Design review of the part built by this model. Coordinates are the model's own, in mm. Face numbers are marked on the shaded views. A direction names the side the tool comes from. Coordinates: 2 decimals unless noted, no trailing zeros. Loops run counter-clockwise (first coordinate to the right, second up) from the corner with the lowest first, then second, coordinate; pieces in that order, holes last. Notation, with made-up numbers: M 36,-38.75 L 77,-38.75 A30 cw 77,-1.75 Z; hole C -36,70.25 d8. An arc over 180 degrees is marked long. Answer as a JSON object with one key per item and string values. Group by question number.
1. Machinability: for the marked faces 5, 6, 7, 8 and 9, which of the approach directions +Z, -Z, +X, -X, +Y, -Y give a long, thin tool a straight path to every point of the face, cutting with its end or side? Answer none if there is none.
2. Consider section D-D (y = 7.75). State the section outline as (x, z) points, then the cut area to 3 significant figures.
3. Consider section C-C (y = 0). Count the separate pieces of the cut face and the enclosed holes in it, then the cut area to 3 significant figures.
4. Consider section B-B (y = -12). State the section outline as (x, z) points, then the cut area to 3 significant figures.
5. Insertion check: pin 1 (2 mm diameter, centred on y = 9.5, z = -20, fed in from +X); pin 2 (1.8 mm diameter, centred on x = -26.5, y = -1.5, fed in from +Z); pin 3 (6.5 mm diameter, centred on x = -1, y = 3.5, fed in from +Z); pin 4 (6.5 mm diameter, centred on x = -27.3, y = 0, fed in from -Z). Each pin has a flat end and moves straight along its axis. Give the tip position at first contact, or say it passes through.
6. Consider section A-A (z = -13.5). State the section outline as (x, y) points, then the cut area to 3 significant figures.
7. To check wall thickness, follow probe 1 along Y at (x, z) = (4, -32.3); probe 2 along Y at (x, z) = (-20, -30.5); probe 3 along Z at (x, y) = (11.7, 0). State the ranges of each line that lie inside material, in increasing order.
8. Draft analysis for pull direction X (two halves, no side actions). For the marked faces 1, 2, 3 and 4, state which applies: +X half, -X half, draft (parallel to the pull), parting line (faces both ways), or undercut.
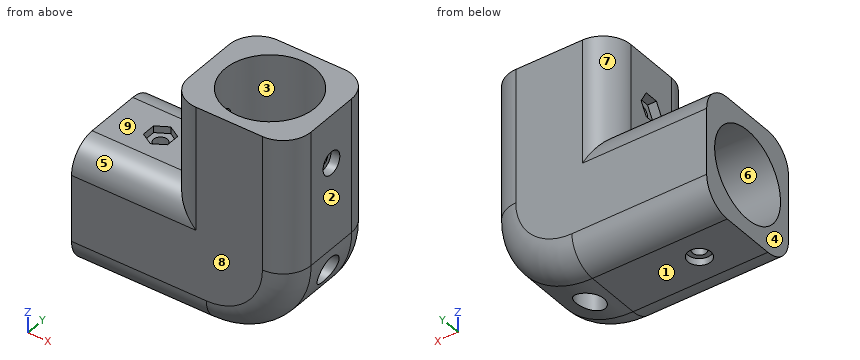
from build123d import *

# Parameters (mm, degrees)
SKETCH1_R           = 13.9
SKETCH1_R_2         = 11.2
BOSS_EXTRUDE1_DEPTH = 7
SKETCH2_W           = 30.6
SKETCH2_H           = 27.8
SKETCH2_R           = 11.2
BOSS_EXTRUDE2_DEPTH = 24
SKETCH6_W           = 30.6
SKETCH6_H           = 27.8
SKETCH6_R           = 11.2
BOSS_EXTRUDE6_DEPTH = 24
SKETCH7_W           = 30.6
SKETCH7_H           = 30.6
BOSS_EXTRUDE7_DEPTH = 27.8
FILLET1_R           = 21
FILLET2_R           = 7
SKETCH8_R           = 3.5
CUT_EXTRUDE1_DEPTH  = 31.6000001
SKETCH9_R           = 3.5
CUT_EXTRUDE2_DEPTH  = 31.6000001
CUT_EXTRUDE3_DEPTH  = 2.2
SKETCH12_R          = 1.7
CUT_EXTRUDE4_DEPTH  = 29.4000001
SKETCH13_R          = 2.85
CUT_EXTRUDE5_DEPTH  = 2.2
CUT_EXTRUDE6_DEPTH  = 1.7
SKETCH16_R          = 1.7
CUT_EXTRUDE7_DEPTH  = 29.9000001
SKETCH17_R          = 2.85
CUT_EXTRUDE8_DEPTH  = 1.7


with BuildPart() as part:
    # Sketch1 → Boss-Extrude1 (new body)
    with BuildSketch(Plane.XY):
        Circle(SKETCH1_R)
        Circle(SKETCH1_R_2, mode=Mode.SUBTRACT)
    extrude(amount=BOSS_EXTRUDE1_DEPTH)

    # Sketch2 → Boss-Extrude2 (add)
    with BuildSketch(Plane.XY.offset(7)):
        Rectangle(SKETCH2_W, SKETCH2_H)
        Circle(SKETCH2_R, mode=Mode.SUBTRACT)
    extrude(amount=-BOSS_EXTRUDE2_DEPTH)



with BuildPart() as body_2:
    # Sketch6 → Boss-Extrude6 (new body)
    with BuildSketch(Plane.ZY.offset(15.3)):
        with Locations((-32.3, 0)):
            Rectangle(SKETCH6_W, SKETCH6_H)
        with Locations((-32.3, 0)):
            Circle(SKETCH6_R, mode=Mode.SUBTRACT)
    extrude(amount=BOSS_EXTRUDE6_DEPTH)


with BuildPart() as part_1:
    add(part.part)

    add(body_2.part)  # Boss-Extrude7 merges body 2
    # Sketch7 → Boss-Extrude7 (add)
    with BuildSketch(Plane(origin=(0, 13.9, 0), x_dir=(1, 0, 0), z_dir=(0, 1, 0))):
        with Locations((0, 32.3)):
            Rectangle(SKETCH7_W, SKETCH7_H)
    extrude(amount=-BOSS_EXTRUDE7_DEPTH)

    # Fillet1
    fillet1_edges = [part_1.edges().sort_by_distance(p)[0] for p in [
        (15.3, 0, -47.6),
    ]]
    fillet(fillet1_edges, radius=FILLET1_R)

    # Fillet2
    fillet2_edges = [part_1.edges().sort_by_distance(p)[0] for p in [
        (-22.5, -13.9, -47.6),
        (-15.3, 13.9, -5),
        (-15.3, -13.9, -5),
        (-27.3, 13.9, -17),
        (-27.3, -13.9, -17),
        (15.3, -13.9, -9.8),
        (15.3, 13.9, -9.8),
        (-22.5, 13.9, -47.6),
        (9.149242405, 13.9, -41.449242405),
        (9.149242405, -13.9, -41.449242405),
    ]]
    fillet(fillet2_edges, radius=FILLET2_R)

    # Sketch8 → Cut-Extrude1 (cut, through all)
    with BuildSketch(Plane.ZY.offset(15.3)):
        with Locations((-32.3, 0)):
            Circle(SKETCH8_R)
    extrude(amount=-CUT_EXTRUDE1_DEPTH, mode=Mode.SUBTRACT)

    # Sketch9 → Cut-Extrude2 (cut, through all)
    with BuildSketch(Plane.XY.offset(-17)):
        Circle(SKETCH9_R)
    extrude(amount=-CUT_EXTRUDE2_DEPTH, mode=Mode.SUBTRACT)

    # Sketch11 → Cut-Extrude3 (cut)
    with BuildSketch(Plane.ZY.offset(15.3)):
        Polygon((-2, -1.732050808), (-2, 1.732050808), (-5, 3.464101615), (-8, 1.732050808), (-8, -1.732050808), (-5, -3.464101615), align=None)
    extrude(amount=-CUT_EXTRUDE3_DEPTH, mode=Mode.SUBTRACT)

    # Sketch12 → Cut-Extrude4 (cut, through all)
    with BuildSketch(Plane.ZY.offset(13.1)):
        with Locations((-5, 0)):
            Circle(SKETCH12_R)
    extrude(amount=-CUT_EXTRUDE4_DEPTH, mode=Mode.SUBTRACT)

    # Sketch13 → Cut-Extrude5 (cut)
    with BuildSketch(Plane(origin=(15.3, 0, 0), x_dir=(0, 0, -1), z_dir=(1, 0, 0))):
        with Locations((5, 0)):
            Circle(SKETCH13_R)
    extrude(amount=-CUT_EXTRUDE5_DEPTH, mode=Mode.SUBTRACT)

    # Sketch15 → Cut-Extrude6 (cut)
    with BuildSketch(Plane.XY.offset(-17)):
        Polygon((-24.3, -1.732050808), (-24.3, 1.732050808), (-27.3, 3.464101615), (-30.3, 1.732050808), (-30.3, -1.732050808), (-27.3, -3.464101615), align=None)
    extrude(amount=-CUT_EXTRUDE6_DEPTH, mode=Mode.SUBTRACT)

    # Sketch16 → Cut-Extrude7 (cut, through all)
    with BuildSketch(Plane.XY.offset(-18.7)):
        with Locations((-27.3, 0)):
            Circle(SKETCH16_R)
    extrude(amount=-CUT_EXTRUDE7_DEPTH, mode=Mode.SUBTRACT)

    # Sketch17 → Cut-Extrude8 (cut)
    with BuildSketch(Plane(origin=(0, 0, -47.6), x_dir=(-1, 0, 0), z_dir=(0, 0, -1))):
        with Locations((27.3, 0)):
            Circle(SKETCH17_R)
    extrude(amount=-CUT_EXTRUDE8_DEPTH, mode=Mode.SUBTRACT)


solid = part_1.part
Findings below:
{
 "1": {"face 5": "+Z, -X, -Y", "face 6": "-X", "face 7": "+Z, -X, +Y", "face 8": "+Z, -Z, +X, -X, -Y", "face 9": "+Z, -X, +Y, -Y"},
 "2": {"outline": "M -39.3,-47.55 L -5.7,-47.55 A20.95 ccw 15.25,-26.6 L 15.25,7 L 8.09,7 L 8.09,-17 L -8.09,-17 L -8.09,7 L -15.25,7 L -15.25,-17.05 L -39.3,-17.05 L -39.3,-24.21 L -15.3,-24.21 L -15.3,-40.39 L -39.3,-40.39 Z", "area": "1,530 mm^2"},
 "3": {"separate pieces": "8", "enclosed holes": "0", "area": "794 mm^2"},
 "4": {"outline": "M -39.3,-45.39 L -5.7,-45.39 A18.79 ccw 13.09,-26.6 L 13.09,7 L -13.09,7 L -13.09,-19.21 L -39.3,-19.21 Z", "area": "1,980 mm^2"},
 "5": {"pin 1": "stops at x = 15.11", "pin 2": "stops at z = -18.7", "pin 3": "stops at z = -17", "pin 4": "stops at z = -47.6"},
 "6": {"outline": "M -15.3,-6.9 A7 ccw -8.3,-13.9 L 8.3,-13.9 A7 ccw 15.3,-6.9 L 15.3,6.9 A7 ccw 8.3,13.9 L -8.3,13.9 A7 ccw -15.3,6.9 Z; hole C 0,0 d22.4", "area": "415 mm^2"},
 "7": {"probe 1": "y = -13.9 to -3.5, 3.5 to 13.9", "probe 2": "y = -13.9 to -11.05, 11.05 to 13.9", "probe 3": "z = -38.36 to -35.8, -28.8 to -6.7, -3.3 to 7"},
 "8": {"face 1": "draft", "face 2": "+X half", "face 3": "undercut", "face 4": "-X half"}
}
